Build history of the part. All positions in model axes, mm. Face numbers are marked on the shaded views. Give positions to 0.01 mm unless a question says otherwise; leave off trailing zeros. Order: outer loops, then holes, each group sorted by start corner. A loop starts at its lowest first (then second) coordinate and runs counter-clockwise, first axis right, second up. Notation, with made-up numbers: (68.25, -34) - (95.25, -34) arc R19 cw to (95.25, -14) - close; hole circle Ø2 at (26.5, 5). An arc over 180 degrees is marked (long way). Use a Markdown table: item, result.
from build123d import *

# Parameters (mm, degrees)
BLANK_OD70_THICKNESS7_MM_W                    = 7
BLANK_OD70_THICKNESS7_MM_H                    = 35
WATER_PASSAGE_R11_25_DEPTH3_ROUND_END_C_DEPTH = 3
INNER_FACE_SEAL_GLAND_WIDTH2P6_DEPTH_2_R      = 9.3
INNER_FACE_SEAL_GLAND_WIDTH2P6_DEPTH_2_R_2    = 6.7
INNER_FACE_SEAL_GLAND_WIDTH2P6_DEPTH1P5_DEPTH = 1.5
OUTER_FACE_SEAL_GLAND_WIDTH2P6_DEPTH_2_R      = 29.3
OUTER_FACE_SEAL_GLAND_WIDTH2P6_DEPTH_2_R_2    = 26.7
OUTER_FACE_SEAL_GLAND_WIDTH2P6_DEPTH1P5_DEPTH = 1.5
SIX_REAR_COVER_M3_PILOT_BORES_DEPTH4_SKE_R    = 1.25
SIX_REAR_COVER_M3_PILOT_BORES_DEPTH4_DEPTH    = 4
THREE_START                                   = 4
THREE_FRONT_CLAMP_M3_PILOT_BORES_DEP_2_R      = 1.25
THREE_FRONT_CLAMP_M3_PILOT_BORES_DEPTH3_DEPTH = 3


with BuildPart() as part:
    # Blank OD70 thickness7 mm → Copper blank - OD70 x7 (revolve)
    with BuildSketch(Plane.XY, mode=Mode.PRIVATE) as copper_blank_od70_x7_sk:
        with Locations((3.5, 17.5)):
            Rectangle(BLANK_OD70_THICKNESS7_MM_W, BLANK_OD70_THICKNESS7_MM_H)
    revolve(copper_blank_od70_x7_sk.sketch.rotate(Axis((-10, 0, 0), (1, 0, 0)), 90), axis=Axis((-10, 0, 0), (1, 0, 0)))

    # Water passage R11-25 depth3 round-en 2 → Water passage R11-25 depth3 round-end C (cut)
    with BuildSketch(Plane(origin=(0, 0, 0), x_dir=(0, 0, -1), z_dir=(1, 0, 0))):
        with BuildLine():
            ThreePointArc((-12.5, 21.650635095), (0, -25), (12.5, 21.650635095))
            ThreePointArc((12.5, 21.650635095), (2.937822174, 19.088457268), (5.5, 9.526279442))
            ThreePointArc((5.5, 9.526279442), (0, -11), (-5.5, 9.526279442))
            ThreePointArc((-5.5, 9.526279442), (-2.937822174, 19.088457268), (-12.5, 21.650635095))
        make_face()
    extrude(amount=WATER_PASSAGE_R11_25_DEPTH3_ROUND_END_C_DEPTH, mode=Mode.SUBTRACT)

    # Inner face-seal gland width2p6 depth 2 → Inner face-seal gland width2p6 depth1p5 (cut)
    with BuildSketch(Plane(origin=(0, 0, 0), x_dir=(0, 0, -1), z_dir=(1, 0, 0))):
        Circle(INNER_FACE_SEAL_GLAND_WIDTH2P6_DEPTH_2_R)
        Circle(INNER_FACE_SEAL_GLAND_WIDTH2P6_DEPTH_2_R_2, mode=Mode.SUBTRACT)
    extrude(amount=INNER_FACE_SEAL_GLAND_WIDTH2P6_DEPTH1P5_DEPTH, mode=Mode.SUBTRACT)

    # Outer face-seal gland width2p6 depth 2 → Outer face-seal gland width2p6 depth1p5 (cut)
    with BuildSketch(Plane(origin=(0, 0, 0), x_dir=(0, 0, -1), z_dir=(1, 0, 0))):
        Circle(OUTER_FACE_SEAL_GLAND_WIDTH2P6_DEPTH_2_R)
        Circle(OUTER_FACE_SEAL_GLAND_WIDTH2P6_DEPTH_2_R_2, mode=Mode.SUBTRACT)
    extrude(amount=OUTER_FACE_SEAL_GLAND_WIDTH2P6_DEPTH1P5_DEPTH, mode=Mode.SUBTRACT)

    # Six rear cover M3 pilot bores depth4 sketch → Six rear cover M3 pilot bores depth4 (cut)
    with BuildSketch(Plane(origin=(0, 0, 0), x_dir=(0, 0, -1), z_dir=(1, 0, 0))):
        with Locations((0, 32)):
            Circle(SIX_REAR_COVER_M3_PILOT_BORES_DEPTH4_SKE_R)
        with Locations((-27.712812921, 16)):
            Circle(SIX_REAR_COVER_M3_PILOT_BORES_DEPTH4_SKE_R)
        with Locations((-27.712812921, -16)):
            Circle(SIX_REAR_COVER_M3_PILOT_BORES_DEPTH4_SKE_R)
        with Locations((0, -32)):
            Circle(SIX_REAR_COVER_M3_PILOT_BORES_DEPTH4_SKE_R)
        with Locations((27.712812921, -16)):
            Circle(SIX_REAR_COVER_M3_PILOT_BORES_DEPTH4_SKE_R)
        with Locations((27.712812921, 16)):
            Circle(SIX_REAR_COVER_M3_PILOT_BORES_DEPTH4_SKE_R)
    extrude(amount=SIX_REAR_COVER_M3_PILOT_BORES_DEPTH4_DEPTH, mode=Mode.SUBTRACT)

    # Three front clamp M3 pilot bores dep 2 → Three front clamp M3 pilot bores depth3 (cut)
    with BuildSketch(Plane(origin=(0, 0, 0), x_dir=(0, 0, -1), z_dir=(1, 0, 0)).offset(THREE_START)):
        with Locations((-16, 27.712812921)):
            Circle(THREE_FRONT_CLAMP_M3_PILOT_BORES_DEP_2_R)
        with Locations((-16, -27.712812921)):
            Circle(THREE_FRONT_CLAMP_M3_PILOT_BORES_DEP_2_R)
        with Locations((32, 0)):
            Circle(THREE_FRONT_CLAMP_M3_PILOT_BORES_DEP_2_R)
    extrude(amount=THREE_FRONT_CLAMP_M3_PILOT_BORES_DEPTH3_DEPTH, mode=Mode.SUBTRACT)


solid = part.part
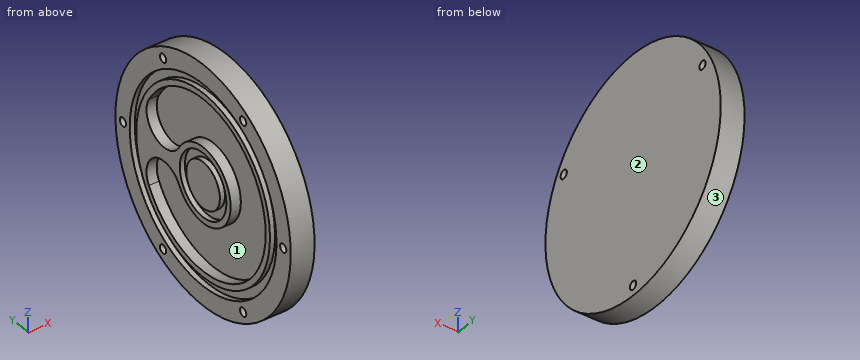
1) Slice it at C-C (x = 6). Write the cut outline in (y, z).
Computed:
| item | result |
|---|---|
| outline | circle Ø70 at (0, 0); hole circle Ø2.5 at (-27.71, 16); hole circle Ø2.5 at (0, -32); hole circle Ø2.5 at (27.71, 16) |
2) Pin check, flat tips, straight feed: P1, Ø1.2, axis at y = 27.5, z = 16, coming from the +X side; P2, Ø1.5, axis at x = 4, y = -23, coming from the -Z side; P3, Ø3, axis at x = 2.5, y = -14, coming from the +Z side. Stop position of each tip, or through.
Computed:
| item | result |
|---|---|
| P1 | stops at x = 4 |
| P2 | stops at z = -27.02 |
| P3 | stops at z = 32.69 |
3) Two-plate mould, pull along Y, no slides. Class the marked faces 1, 2 and 3: +Y half, -Y half, draft (parallel to the pull), parting line (faces both ways), or undercut.
Computed:
| item | result |
|---|---|
| face 1 | undercut |
| face 2 | draft |
| face 3 | parting line |
4) Slice it at D-D (z = -32). Write the cut outline in (x, y), and give its area (3 significant figures).
Computed:
| item | result |
|---|---|
| outline | (0, -14.18) - (7, -14.18) - (7, -1.25) - (4, -1.25) - (4, 1.25) - (7, 1.25) - (7, 14.18) - (0, 14.18) - close |
| area | 191 mm² |
5) Slice it at B-B (y = 3.5). Write the cut outline in (x, z), and give its area (3 significant figures).
Computed:
| item | result |
|---|---|
| outline | (0, -34.82) - (7, -34.82) - (7, 34.82) - (0, 34.82) - (0, 29.09) - (1.5, 29.09) - (1.5, 26.47) - (0, 26.47) - (0, 24.75) - (3, 24.75) - (3, 10.43) - (0, 10.43) - (0, 8.62) - (1.5, 8.62) - (1.5, 5.71) - (0, 5.71) - (0, -5.71) - (1.5, -5.71) - (1.5, -8.62) - (0, -8.62) - (0, -10.43) - (3, -10.43) - (3, -24.75) - (0, -24.75) - (0, -26.47) - (1.5, -26.47) - (1.5, -29.09) - (0, -29.09) - close |
| area | 385 mm² |
6) Wall check: line 1 (Z direction, x = 2.5, y = -17); line 2 (Y direction, x = 2.5, z = 27); line 3 (Z direction, x = 2.5, y = 5.5). Give the ranges that are in metal, low to high. Write a range as from..to.
Computed:
| item | result |
|---|---|
| line 1 | z = -30.59..-28.46, -26.96..-18.33, 18.33..26.96, 28.46..30.59 |
| line 2 | y = -22.27..-17.03, -14.97..14.97, 17.03..22.27 |
| line 3 | z = -34.57..-24.39, -9.53..9.53, 24.39..34.57 |
